from build123d import *

# Parameters (mm, degrees)
EXTRUDE_1_DEPTH     = 9
SKETCH_2_R          = 3.5
CUT_EXTRUDE_1_DEPTH = 18
EXTRUDE_2_DEPTH     = 10
EXTRUDE_START       = 2.5
SKETCH_4_R          = 3.5
EXTRUDE_3_DEPTH     = 2.5
CHAMFER_1_SIZE      = 1
EXTRUDE_4_DEPTH     = 10
SKETCH_7_W          = 63.046601733
SKETCH_7_H          = 81.446187988
CUT_EXTRUDE_2_DEPTH = 10
SKETCH_8_W          = 55.396674472
SKETCH_8_H          = 20
EXTRUDE_5_DEPTH     = 2


with BuildPart() as part:
    # 草图1 → 凸台-拉伸1 (new, symmetric)
    with BuildSketch(Plane.XY):
        with BuildLine():
            Line((-38.810889132, -2.777568136), (-8.5, 14.722431864))
            ThreePointArc((-8.5, 14.722431864), (-1.481647627, 16.935309868), (5.814342437, 15.974774553))
            Line((5.814342437, 15.974774553), (6.498382723, 17.854159795))
            ThreePointArc((6.498382723, 17.854159795), (-1.655959112, 18.927699264), (-9.5, 16.454482672))
            Line((-9.5, 16.454482672), (-39.810889132, -1.045517328))
            Line((-39.810889132, -1.045517328), (-38.810889132, -2.777568136))
        make_face()
    extrude(amount=EXTRUDE_1_DEPTH, both=True)

    # 草图2 → 切除-拉伸1 (cut)
    with BuildSketch(Plane(origin=(-9.5, 16.454482672, 0), x_dir=(0.8660254037844398, 0.49999999999999806, 0), z_dir=(-0.49999999999999806, 0.8660254037844398, 0))):
        with Locations(Location((-26, 0, 0), (0, 0, 180))):
            Circle(SKETCH_2_R)
    extrude(amount=-CUT_EXTRUDE_1_DEPTH, mode=Mode.SUBTRACT)

    # 草图7 → 切除-拉伸2 (cut, symmetric)
    with BuildSketch(Plane.XY):
        with Locations((-23.889592718, 14.899687111)):
            Rectangle(SKETCH_7_W, SKETCH_7_H)
    extrude(amount=CUT_EXTRUDE_2_DEPTH, both=True, mode=Mode.SUBTRACT)


with BuildPart() as body_2:
    # 草图3 → 凸台-拉伸2 (new, symmetric)
    with BuildSketch(Plane.XY):
        Polygon((-26.266761163, 4.464787524), (-69.318063007, -30.397469317), (-71.206024181, -28.066031433), (-42.87484181, -5.123892308), align=None)
    extrude(amount=EXTRUDE_2_DEPTH, both=True)

    # 草图4 → 凸台-拉伸3 (add)
    with BuildSketch(Plane(origin=(-8.5, 14.722431864, 0), x_dir=(0.8660254037844386, 0.5000000000000001, 0), z_dir=(-0.5000000000000001, 0.8660254037844386, 0)).offset(EXTRUDE_START)):
        with Locations((-26, 0)):
            Circle(SKETCH_4_R)
    extrude(amount=-EXTRUDE_3_DEPTH)

    # 倒角1
    chamfer_1_edges = [body_2.edges().sort_by_distance(p)[0] for p in [
        (-35.297749412, 2.137495374, 0),
    ]]
    chamfer(chamfer_1_edges, length=CHAMFER_1_SIZE)

    # 草图6 → 凸台-拉伸4 (add, symmetric)
    with BuildSketch(Plane.XY):
        Polygon((-38.810889132, -2.777568136), (-39.182510373, -2.133901265), (-42.87484181, -5.123892308), align=None)
    extrude(amount=EXTRUDE_4_DEPTH, both=True)

    # 草图8 → 凸台-拉伸5 (add)
    with BuildSketch(Plane(origin=(-12.586407821, 15.542919229, 0), x_dir=(0.7771459614569706, 0.6293203910498378, 0), z_dir=(0.6293203910498378, -0.7771459614569706, 0))):
        with Locations((-45.301662764, 0)):
            Rectangle(SKETCH_8_W, SKETCH_8_H)
    extrude(amount=EXTRUDE_5_DEPTH)


solid = body_2.part
Design review of the part built by this model. Coordinates are the model's own, in mm. Round coordinates to 2 decimals unless told otherwise and drop trailing zeros. Order: outer loops, then holes, each group sorted by start corner. A loop starts at its lowest first (then second) coordinate and runs counter-clockwise, first axis right, second up.
1) Draft analysis for pull direction X (two halves, no side actions). For faces 1 (the cylindrical face through (-28.6, 4, 1.34)), 2 (the flat face through (-46.835, -14.765, 0.14)), 3 (the flat face through (-48, -13, -10)), state which applies: released by +X, released by -X, zero draft, split by the parting line, or undercut.
The answers:
face 1: undercut
face 2: released by +X
face 3: zero draft
2) Consider section C-C (x = -35.5). State the section outline as (y, z) points.
The answers:
outline: (-5.59, -10) - (-0.87, -10) - (-0.87, 10) - (-5.59, 10) - close
3) For L1, parallel to X at y = -11.5, z = 5.75; L2, parallel to X at y = -25.5, z = 7; L3, parallel to Y at x = -45, z = -3.25, list the stretches that pass through material, from the lowest coordinate up.
The answers:
L1: x = -50.75 to -42.8
L2: x = -68.04 to -60.09
L3: y = -13.28 to -6.84
4) Consider section A-A (z = 6.75). State the section outline as (x, y) points.
The answers:
outline: (-71.21, -28.07) - (-68.06, -31.95) - (-25.01, 2.91) - (-26.27, 4.46) - (-38.81, -2.78) - (-39.18, -2.13) - close
5) Consider section B-B (y = -29). State the section outline as (x, z) points, plus the area to 3 significant figures.
The answers:
outline: (-70.45, -10) - (-64.41, -10) - (-64.41, 10) - (-70.45, 10) - close
area: 121 mm2
6) Clearance check with flat-ended pins moving along their axes: pin 1 Ø8 at (x, z) = (-45.5, 5.5) entering from +Y; pin 2 Ø8 at (y, z) = (0, -5) entering from +X; pin 3 Ø6 at (x, z) = (-55, 1) entering from +Y; pin 4 Ø10 at (x, y) = (-65.5, -13) entering from -Z. State where each tip first meets the part, or that it passes through.
The answers:
pin 1: stops at y = -4.01
pin 2: stops at x = -25.01
pin 3: stops at y = -12.51
pin 4: passes through
